Geometry check sheet. Reference: the model listing, model coordinates, mm. Coordinates: 2 decimals unless noted, no trailing zeros. Loops run counter-clockwise (first coordinate to the right, second up) from the corner with the lowest first, then second, coordinate; pieces in that order, holes last.
from build123d import *

# Parameters (mm, degrees)
F1_DEPTH    = 25.4
F2_DEPTH    = 25.4
F3_T1_DEPTH = 60.9890887747


# Not quite as in the source:
# - a fillet or chamfer that OpenCascade refuses, or shapes differently, is made with other operations: its cross-section is extruded or revolved along the edge and cut away or added


with BuildPart() as f1:
    # F0 (on Top) → F1 (new body)
    with BuildSketch(Plane.XY):
        with BuildLine():
            Line((0, 0), (9.0822612578, 0))
            add(Edge.make_bspline(
                [(9.0822612578, 0), (-0.5887823283, 1.5524321895), (-10.1972217153, 3.0991138841), (-19.7038336111, 4.636442237)],
                knots=[0.053890232, 0.053890232, 0.053890232, 0.053890232, 0.0876539783, 0.0876539783, 0.0876539783, 0.0876539783], degree=3))
            Line((-19.7038336111, 4.636442237), (-18.3546670651, 0.4999203421))
            Line((-18.3546670651, 0.4999203421), (-18.4854740521, 0))
            Line((-18.4854740521, 0), (0, 0))
        make_face()
    extrude(amount=F1_DEPTH)

    # F0 (on Top) → F2 (join)
    with BuildSketch(Plane.XY):
        with BuildLine():
            ThreePointArc((39.2946183394, 19.5425995517), (38.0990536847, 9.5917687024), (35.1927875929, 0))
            ThreePointArc((35.1927875929, 0), (35.1315324061, -2.0755070121), (34.9479800825, -4.1437889318))
            add(Edge.make_bspline(
                [(53.7340444048, -7.1471543317), (47.4674866948, -6.1456158537), (41.202016032, -5.1441772263), (34.9479800825, -4.1437889318)],
                knots=[0.0022748674, 0.0022748674, 0.0022748674, 0.0022748674, 0.0239294634, 0.0239294634, 0.0239294634, 0.0239294634], degree=3))
            Line((53.7340444048, -7.1471543317), (54.1296049181, -6.5938649088))
            Line((54.1296049181, -6.5938649088), (54.6883645828, 4.6909042491))
            Line((54.6883645828, 4.6909042491), (49.0574163024, 14.4863444523))
            Line((49.0574163024, 14.4863444523), (39.2946183394, 19.5425995517))
        make_face()
        with BuildLine():
            ThreePointArc((29.7418780254, 18.8136384064), (33.8026026699, 9.793689361), (35.1927875929, 0))
            ThreePointArc((35.1927875929, 0), (38.0990536847, 9.5917687024), (39.2946183394, 19.5425995517))
            Line((39.2946183394, 19.5425995517), (39.0245463695, 19.6824726475))
            Line((39.0245463695, 19.6824726475), (29.7418780254, 18.8136384064))
        make_face()
        with BuildLine():
            ThreePointArc((-31.426870984, 15.839320652), (-1.7092225846, 35.1512568298), (29.7418780254, 18.8136384064))
            Line((29.7418780254, 18.8136384064), (39.0245463695, 19.6824726475))
            Line((39.0245463695, 19.6824726475), (39.2946183394, 19.5425995517))
            ThreePointArc((39.2946183394, 19.5425995517), (29.0039385515, 54.2539705519), (0, 75.9230479598))
            ThreePointArc((0, 75.9230479598), (-13.7345779986, 68.6878764709), (-25.1210674885, 58.1363743803))
            ThreePointArc((-25.1210674885, 58.1363743803), (-35.8950760367, 38.527599561), (-38.637588859, 16.3226016208))
            Line((-38.637588859, 16.3226016208), (-38.0839338665, 16.5955866568))
            Line((-38.0839338665, 16.5955866568), (-31.426870984, 15.839320652))
        make_face()
        with BuildLine():
            add(Edge.make_bspline(
                [(53.7340444048, -7.1471543317), (47.4674866948, -6.1456158537), (41.202016032, -5.1441772263), (34.9479800825, -4.1437889318)],
                knots=[0.0022748674, 0.0022748674, 0.0022748674, 0.0022748674, 0.0239294634, 0.0239294634, 0.0239294634, 0.0239294634], degree=3))
            ThreePointArc((34.9479800825, -4.1437889318), (33.2140769684, -11.6343194773), (29.8948841627, -18.56955033))
            Line((29.8948841627, -18.56955033), (37.0614353142, -19.964725406))
            Line((37.0614353142, -19.964725406), (47.5585395538, -15.7851285483))
            Line((47.5585395538, -15.7851285483), (53.7340444048, -7.1471543317))
        make_face()
        with BuildLine():
            ThreePointArc((29.8948841627, -18.56955033), (33.2140769684, -11.6343194773), (34.9479800825, -4.1437889318))
            add(Edge.make_bspline(
                [(34.9479800825, -4.1437889318), (28.5019841788, -3.1126949471), (22.0681357101, -2.0827167623), (15.6577647144, -1.0548950957)],
                knots=[0.0239294634, 0.0239294634, 0.0239294634, 0.0239294634, 0.0462487206, 0.0462487206, 0.0462487206, 0.0462487206], degree=3))
            Line((15.6577647144, -1.0548950956), (17.8084989026, -9.9934284194))
            Line((17.8084989026, -9.9934284194), (25.9710486263, -17.8056630113))
            Line((25.9710486263, -17.8056630113), (29.8948841627, -18.56955033))
        make_face()
        with BuildLine():
            ThreePointArc((-31.4678779331, -15.7576951661), (-1.6109654608, -35.1558969285), (29.8948841627, -18.56955033))
            Line((29.8948841627, -18.56955033), (25.9710486263, -17.8056630113))
            Line((25.9710486263, -17.8056630113), (17.8084989026, -9.9934284194))
            Line((17.8084989026, -9.9934284194), (15.6577647144, -1.0548950956))
            add(Edge.make_bspline(
                [(15.6577647144, -1.0548950957), (13.4630266479, -0.7029966893), (11.271040594, -0.3513510685), (9.0822612578, 0)],
                knots=[0.0462487206, 0.0462487206, 0.0462487206, 0.0462487206, 0.053890232, 0.053890232, 0.053890232, 0.053890232], degree=3))
            Line((9.0822612578, 0), (0, 0))
            Line((0, 0), (-18.4854740521, 0))
            Line((-18.4854740521, 0), (-20.7573818702, -8.6828154927))
            Line((-20.7573818702, -8.6828154927), (-27.7432359966, -15.1088187584))
            Line((-27.7432359966, -15.1088187584), (-31.4678779331, -15.7576951661))
        make_face()
        with BuildLine():
            Line((-37.0942701188, -16.7378788221), (-31.4678779331, -15.7576951661))
            ThreePointArc((-31.4678779331, -15.7576951661), (-34.2489024836, -8.0959852539), (-35.1927875929, 0))
            ThreePointArc((-35.1927875929, 0), (-36.4082086965, 3.7156215634), (-37.3761939959, 7.5032456896))
            add(Edge.make_bspline(
                [(-37.3761939959, 7.5032456896), (-41.0895221285, 8.1076779871), (-44.782988486, 8.7102858856), (-48.4541472769, 9.3108447276)],
                knots=[0.1087279171, 0.1087279171, 0.1087279171, 0.1087279171, 0.1221167407, 0.1221167407, 0.1221167407, 0.1221167407], degree=3))
            Line((-48.4541472769, 9.3108447276), (-51.4896897645, 4.2641766931))
            Line((-51.4896897645, 4.2641766931), (-51.2080020921, -5.2235168043))
            Line((-51.2080020921, -5.2235168043), (-45.8415969743, -13.052780624))
            Line((-45.8415969743, -13.052780624), (-37.0942701188, -16.7378788221))
        make_face()
        with BuildLine():
            ThreePointArc((-35.1927875929, 0), (-34.2489024836, -8.0959852539), (-31.4678779331, -15.7576951661))
            Line((-31.4678779331, -15.7576951661), (-27.7432359966, -15.1088187584))
            Line((-27.7432359966, -15.1088187584), (-20.7573818702, -8.6828154927))
            Line((-20.7573818702, -8.6828154927), (-18.4854740521, 0))
            Line((-18.4854740521, 0), (-35.1927875929, 0))
        make_face()
        with BuildLine():
            ThreePointArc((-38.637588859, 16.3226016208), (-35.8950760367, 38.527599561), (-25.1210674885, 58.1363743803))
            add(Edge.make_bspline(
                [(-48.4541472769, 9.3108447276), (-161.5048500043, 27.8046236609), (-354.0298848729, 62.4785632102), (-140.2321873005, 59.829817618), (-25.1210674885, 58.1363743803)],
                knots=[0.1221167407, 0.1221167407, 0.1221167407, 0.1221167407, 0.5344159633, 0.9858900342, 0.9858900342, 0.9858900342, 0.9858900342], degree=3))
            Line((-48.4541472769, 9.3108447276), (-46.5972261458, 12.3980242197))
            Line((-46.5972261458, 12.3980242197), (-38.637588859, 16.3226016208))
        make_face()
        with BuildLine():
            add(Edge.make_bspline(
                [(-37.3761939959, 7.5032456896), (-41.0895221285, 8.1076779871), (-44.782988486, 8.7102858856), (-48.4541472769, 9.3108447276)],
                knots=[0.1087279171, 0.1087279171, 0.1087279171, 0.1087279171, 0.1221167407, 0.1221167407, 0.1221167407, 0.1221167407], degree=3))
            ThreePointArc((-37.3761939959, 7.5032456896), (-38.172734201, 11.8892038706), (-38.637588859, 16.3226016208))
            Line((-38.637588859, 16.3226016208), (-46.5972261458, 12.3980242197))
            Line((-46.5972261458, 12.3980242197), (-48.4541472769, 9.3108447276))
        make_face()
    extrude(amount=F2_DEPTH)

    # F3: chamfer of 5.08 on 1 edges, made by hand

    # F3_s2 → F3_t1 (cut)
    with BuildSketch(Plane.XY.offset(-17.7945443873)):
        with BuildLine():
            Line((6.6348201683, 73.3457449263), (-6.5209439135, 73.161183328))
            Line((-6.5209439135, 73.161183328), (-6.5669480575, 73.2517712893))
            ThreePointArc((-6.5669480575, 73.2517712893), (-3.3257137482, 74.6908686941), (-0.0351808653, 76.018362527))
            Line((-0.0351808653, 76.018362527), (0.0320735811, 76.019452552))
            ThreePointArc((0.0320735811, 76.019452552), (3.3798158566, 74.7892252054), (6.6782649991, 73.4375877631))
            Line((6.6782649991, 73.4375877631), (6.6348201683, 73.3457449263))
        make_face()
    extrude(amount=F3_T1_DEPTH, mode=Mode.SUBTRACT)


solid = f1.part
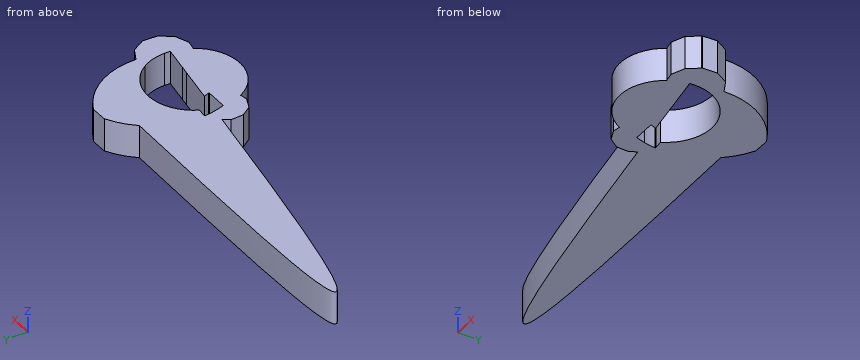
1) Material ranges on probe 1 along Y at (x, z) = (-31, 18.25); probe 2 along Y at (x, z) = (-27.5, 3.25); probe 3 along X at (y, z) = (7, 9.25), recorded low to high.
Data:
probe 1: y = -16.66 to 0, 16.66 to 58.22
probe 2: y = -21.96 to 0, 21.96 to 58.17
probe 3: x = -49.84 to -37.26, 34.49 to 53.36
2) Section check A-A on y = -24.5. Record the cut outline in (x, z), and give its area (3 significant figures).
Data:
outline: (-25.26, 0) - (25.26, 0) - (25.26, 25.4) - (-25.26, 25.4) - close
area: 1,280 mm2
3) Depth check by flat-ended pin: pin 1 (1.5 mm diameter, centred on y = 57, z = 20, fed in from +X); pin 2 (1.5 mm diameter, centred on x = -49.5, z = 10, fed in from -Y); pin 3 (8.5 mm diameter, centred on x = -24, z = 9, fed in from +Y). Enter the tip coordinate at first touch or a pass-through.
Data:
pin 1: stops at x = 27.55
pin 2: stops at y = -8.81
pin 3: stops at y = 63.81
